Model file for the job. Use its own axes, mm. A direction names the side the tool comes from. Give positions to 0.01 mm unless a question says otherwise; leave off trailing zeros. Loops run counter-clockwise (first coordinate to the right, second up) from the corner with the lowest first, then second, coordinate; pieces in that order, holes last. Notation, with made-up numbers: M -20.75,71.5 L -1.75,71.5 A15 ccw -1.75,86.5 Z; hole C 33,-21 d11. An arc over 180 degrees is marked long. Answer in a Markdown table with one row per item.
```python
from build123d import *

# Parameters (mm, degrees)
CROQUIS1_R              = 4
SALIENTE_EXTRUIR1_DEPTH = 3
CROQUIS2_W              = 183.661988175
CROQUIS2_H              = 35
CORTAR_EXTRUIR1_DEPTH   = 4


with BuildPart() as part:
    # Croquis1 → Saliente-Extruir1 (new body)
    with BuildSketch(Plane.XY):
        Polygon((-84, 37.295390898), (-87.2, 37.295390898), (-87.2, 22.295390898), (-84, 22.295390898), (-84, 11.147890898), (-87.2, 11.147890898), (-87.2, -10.945390898), (-84, -10.945390898), (-84, -22.295390898), (-87.2, -22.295390898), (-87.2, -37.295390898), (-84, -37.295390898), (-84, -50), (84, -50), (84, -37.295390898), (87.2, -37.295390898), (87.2, -22.295390898), (84, -22.295390898), (84, -10.945390898), (87.2, -10.945390898), (87.2, 11.147890898), (84, 11.147890898), (84, 22.295390898), (87.2, 22.295390898), (87.2, 37.295390898), (84, 37.295390898), (84, 50), (-84, 50), align=None)
        Circle(CROQUIS1_R, mode=Mode.SUBTRACT)
        with BuildLine():
            Line((-75, -25), (75, -25))
            ThreePointArc((75, -25), (80, -30), (75, -35))
            Line((75, -35), (-75, -35))
            ThreePointArc((-75, -35), (-80, -30), (-75, -25))
        make_face(mode=Mode.SUBTRACT)
        with BuildLine():
            Line((-75, 25), (75, 25))
            ThreePointArc((75, 25), (80, 30), (75, 35))
            Line((75, 35), (-75, 35))
            ThreePointArc((-75, 35), (-80, 30), (-75, 25))
        make_face(mode=Mode.SUBTRACT)
    extrude(amount=SALIENTE_EXTRUIR1_DEPTH)

    # Croquis2 → Cortar-Extruir1 (cut, through all)
    with BuildSketch(Plane.XY.offset(3)):
        with Locations((-0.5645348, 32.5)):
            Rectangle(CROQUIS2_W, CROQUIS2_H)
    extrude(amount=-CORTAR_EXTRUIR1_DEPTH, mode=Mode.SUBTRACT)


solid = part.part
```
(1) Flat gauge pins, fed straight in: P1, Ø0.9, axis at y = 14, z = 2, coming from the +X side; P2, Ø1.5, axis at x = -85, z = 2, coming from the +Y side; P3, Ø0.9, axis at x = 86, z = 1.5, coming from the -Y side; P4, Ø5, axis at x = 0, y = 0, coming from the +Z side. Where does each tip first touch, or does it go through?
Established:
| item | result |
|---|---|
| P1 | stops at x = 84 |
| P2 | stops at y = 11.15 |
| P3 | stops at y = -37.3 |
| P4 | passes through |
(2) Which spindle directions (+Z, -Z, +X, -X, +Y, -Y) get a long thin tool onto all of the face, cutting with end or side? Do faces 4 (the cylindrical face through (80, -30, 1)), 5 (the flat face through (84, -17, 1)), 6 (the flat face through (-86, -22.295, 1)), 7 (the flat face through (84, 13, 1)). Say none if no direction does.
Established:
| item | result |
|---|---|
| face 4 | +Z, -Z |
| face 5 | +Z, -Z, +X |
| face 6 | +Z, -Z, -X |
| face 7 | +Z, -Z, +X, +Y |
(3) Mould opens along Y. For faces 1 (the flat face through (-1, -25, 1)), 2 (the flat face through (-84, -44, 1)), 3 (the flat face through (-86, -37.295, 1)) say: pulls with the +Y half, pulls with the -Y half, needs draft (parallel to the pull), parting line crosses it, or undercut.
Established:
| item | result |
|---|---|
| face 1 | undercut |
| face 2 | needs draft |
| face 3 | pulls with the -Y half |
(4) Saw through at C-C, the plane z = 1.8. Give the cut face in (x, y), and give its area (3 significant figures).
Established:
| item | result |
|---|---|
| outline | M -87.2,-37.3 L -84,-37.3 L -84,-50 L 84,-50 L 84,-37.3 L 87.2,-37.3 L 87.2,-22.3 L 84,-22.3 L 84,-10.95 L 87.2,-10.95 L 87.2,11.15 L 84,11.15 L 84,15 L -84,15 L -84,11.15 L -87.2,11.15 L -87.2,-10.95 L -84,-10.95 L -84,-22.3 L -87.2,-22.3 Z; hole M -75,-35 L 75,-35 A5 ccw 75,-25 L -75,-25 A5 ccw Z; hole C 0,0 d8 |
| area | 9,530 mm2 |
(5) Saw through at B-B, the plane x = -26. Give the cut face in (y, z).
Established:
| item | result |
|---|---|
| outline | M -50,0 L -35,0 L -35,3 L -50,3 Z; M -25,0 L 15,0 L 15,3 L -25,3 Z |
(6) Saw through at A-A, the plane y = 0. Give the cut face in (x, z), and give its area (3 significant figures).
Established:
| item | result |
|---|---|
| outline | M -87.2,0 L -4,0 L -4,3 L -87.2,3 Z; M 4,0 L 87.2,0 L 87.2,3 L 4,3 Z |
| area | 499 mm2 |
(7) Saw through at D-D, the plane x = 0. Give the cut face in (y, z).
Established:
| item | result |
|---|---|
| outline | M -50,0 L -35,0 L -35,3 L -50,3 Z; M -25,0 L -4,0 L -4,3 L -25,3 Z; M 4,0 L 15,0 L 15,3 L 4,3 Z |
(8) Wall check: L1, parallel to Y at x = 0, z = 0.85; L2, parallel to Y at x = 14, z = 1.45; L3, parallel to X at y = -17, z = 0.75. Give the ranges that are in metal, low to high.
Established:
| item | result |
|---|---|
| L1 | y = -50 to -35, -25 to -4, 4 to 15 |
| L2 | y = -50 to -35, -25 to 15 |
| L3 | x = -84 to 84 |
